```python
from build123d import *

# Parameters (mm, degrees)
SKETCH1_R           = 3.175
BOSS_EXTRUDE1_DEPTH = 2.54
CUTOUTS_R           = 11.1125
CUTOUTS_R_2         = 4.572
CUTOUTS_W           = 22.987
CUTOUTS_H           = 17.145
CUTOUTS_R_3         = 1.63195
CUTOUTS_W_2         = 245.872
CUTOUTS_H_2         = 159.512
CUTOUTS_R_4         = 1.905
CUTOUTS_R_5         = 1.2446
CUTOUTS_R_6         = 1.2192
CUTOUTS_R_7         = 2.159
CUTOUTS_R_8         = 39.6875
CUT_EXTRUDE2_DEPTH  = 2.54


with BuildPart() as part:
    # Sketch1 → Boss-Extrude1 (new body)
    with BuildSketch(Plane.XY):
        with BuildLine():
            Line((12.466633151, -16.004721173), (-220.895866849, -16.004721173))
            Line((-220.895866849, -16.004721173), (-220.895866849, 75.745957455))
            add(Edge.make_bspline(
                [(238.947265279, 225.295278827), (159.185673744, 225.799300987), (43.873806561, 224.990313445), (-86.64121676, 195.723193048), (-170.078039566, 157.179815606), (-220.832811132, 123.612518821), (-220.895866849, 75.745957455)],
                knots=[0, 0, 0, 0, 0.46349441, 0.667883071, 0.767851209, 1, 1, 1, 1], degree=3))
            Line((238.947265279, 225.295278827), (238.947265279, -16.004721173))
            Line((238.947265279, -16.004721173), (58.186633151, -16.004721173))
            ThreePointArc((58.186633151, -16.004721173), (35.326633151, 0.432794328), (12.466633151, -16.004721173))
        make_face()
        with Locations((8.951187051, -7.800096672)):
            Circle(SKETCH1_R, mode=Mode.SUBTRACT)
    extrude(amount=BOSS_EXTRUDE1_DEPTH)

    # Cutouts → Cut-Extrude2 (cut)
    with BuildSketch(Plane.XY.offset(2.54)):
        with Locations((-83.250919967, 150.449868461)):
            Circle(CUTOUTS_R)
        with Locations((33.209986811, 195.753851713)):
            Circle(CUTOUTS_R_2)
        with Locations((71.309986811, 195.753851713)):
            Circle(CUTOUTS_R_2)
        with Locations((173.460984528, 198.334802895)):
            Rectangle(CUTOUTS_W, CUTOUTS_H)
        with Locations((158.957584528, 198.612997235)):
            Circle(CUTOUTS_R_3)
        with Locations((187.964384528, 198.612997235)):
            Circle(CUTOUTS_R_3)
        with Locations((79.716556409, 101.851278827)):
            Rectangle(CUTOUTS_W_2, CUTOUTS_H_2)
        with Locations((-47.283443591, 170.177278827)):
            Circle(CUTOUTS_R_4)
        with Locations((-47.283443591, 164.627278827)):
            Circle(CUTOUTS_R_5)
        with Locations((-47.283443591, 45.209278827)):
            Circle(CUTOUTS_R_4)
        with Locations((-47.283443591, 39.659278827)):
            Circle(CUTOUTS_R_5)
        with Locations((206.716556409, 45.209278827)):
            Circle(CUTOUTS_R_4)
        with Locations((206.716556409, 39.659278827)):
            Circle(CUTOUTS_R_5)
        with Locations((206.716556409, 170.177278827)):
            Circle(CUTOUTS_R_4)
        with Locations((-47.283443591, 175.727278827)):
            Circle(CUTOUTS_R_5)
        with Locations((-47.283443591, 50.759278827)):
            Circle(CUTOUTS_R_5)
        with Locations((206.716556409, 175.727278827)):
            Circle(CUTOUTS_R_5)
        with Locations((206.716556409, 164.627278827)):
            Circle(CUTOUTS_R_5)
        with Locations((206.716556409, 50.759278827)):
            Circle(CUTOUTS_R_5)
        Polygon((-95.799367816, 2.039302847), (-95.799367816, 33.535302847), (-111.039367816, 33.535302847), (-111.039367816, 38.361302847), (-165.903367816, 38.361302847), (-165.903367816, 33.535302847), (-181.143367816, 33.535302847), (-181.143367816, 2.039302847), (-165.903367816, 2.039302847), (-165.903367816, -2.786697153), (-111.039367816, -2.786697153), (-111.039367816, 2.039302847), align=None)
        with Locations((-169.865767816, 36.837302847)):
            Circle(CUTOUTS_R_4)
        with Locations((-107.076967816, -1.262697153)):
            Circle(CUTOUTS_R_4)
        with Locations((-107.076967816, 36.837302847)):
            Circle(CUTOUTS_R_4)
        with Locations((-175.402967816, 36.837302847)):
            Circle(CUTOUTS_R_6)
        with Locations((-180.965567816, 36.837302847)):
            Circle(CUTOUTS_R_6)
        with Locations((-169.865767816, -1.262697153)):
            Circle(CUTOUTS_R_4)
        with Locations((-175.402967816, -1.262697153)):
            Circle(CUTOUTS_R_6)
        with Locations((-180.965567816, -1.262697153)):
            Circle(CUTOUTS_R_6)
        with Locations((-101.539767816, -1.262697153)):
            Circle(CUTOUTS_R_6)
        with Locations((-95.977167816, -1.262697153)):
            Circle(CUTOUTS_R_6)
        with Locations((-101.539767816, 36.837302847)):
            Circle(CUTOUTS_R_6)
        with Locations((-95.977167816, 36.837302847)):
            Circle(CUTOUTS_R_6)
        with Locations((-103.103366849, 57.972778827)):
            Circle(CUTOUTS_R_7)
        with Locations((-134.535866849, 89.405278827)):
            Circle(CUTOUTS_R_8)
        with Locations((-165.968366849, 57.972778827)):
            Circle(CUTOUTS_R_7)
        with Locations((-103.103366849, 120.837778827)):
            Circle(CUTOUTS_R_7)
        with Locations((-165.968366849, 120.837778827)):
            Circle(CUTOUTS_R_7)
    extrude(amount=-CUT_EXTRUDE2_DEPTH, mode=Mode.SUBTRACT)


solid = part.part
```
Input: part model. Units: mm. Frame: model coordinates. Coordinates: 2 decimals unless noted, no trailing zeros. Answer as a JSON object with one key per item and string values.
1. First-contact query: P1, Ø5.5, axis at x = 33.21, y = 195.75, coming from the -Z side. Flat tip, straight axial feed; report the tip coordinate or a pass-through.
Result set:
{"P1": "passes through"}
2. Material intervals for line 1 (X direction, y = 45, z = 0.25); line 2 (X direction, y = 25, z = 1.4); line 3 (Y direction, x = 171, z = 1.95), sorted ascending. Write a range as from..to.
Result set:
{"line 1": "x = -220.9..-49.18, -45.39..-43.22, 202.65..204.82, 208.61..238.95", "line 2": "x = -220.9..-181.14, -95.8..-43.22, 202.65..238.95", "line 3": "y = -16..22.1, 181.61..189.76, 206.91..225.22"}
3. Section A-A on y = 106.5. Count the separate pieces of the cut face and the enclosed holes in it, then the cut area to 3 significant figures.
Result set:
{"separate pieces": "3", "enclosed holes": "0", "area": "347 mm2"}
4. Mould query, pull axis Y, two halves, no side actions, for faces 1 (the face through (66.742, 195.955, 1.288)), 2 (the face through (12, 187, 0)), 3 (the face through (35.75, 0.43, 1.25)). Classes: released by +Y, released by -Y, zero draft, split by the parting line, or undercut.
Result set:
{"face 1": "undercut", "face 2": "zero draft", "face 3": "released by -Y"}
